Could you check a few things on this drawing? It's one solid part, dimensions in mm from its lowest x, y, z. A direction names the side the tool comes from. Round coordinates to 2 decimals unless told otherwise and drop trailing zeros. Loops run counter-clockwise (first coordinate to the right, second up) from the corner with the lowest first, then second, coordinate; pieces in that order, holes last. Notation, with made-up numbers: M 4,55 L 9,55 A6 ccw 9,66 Z; hole C 74,-35 d8. An arc over 180 degrees is marked long. Answer as a JSON object with one key per item and string values.
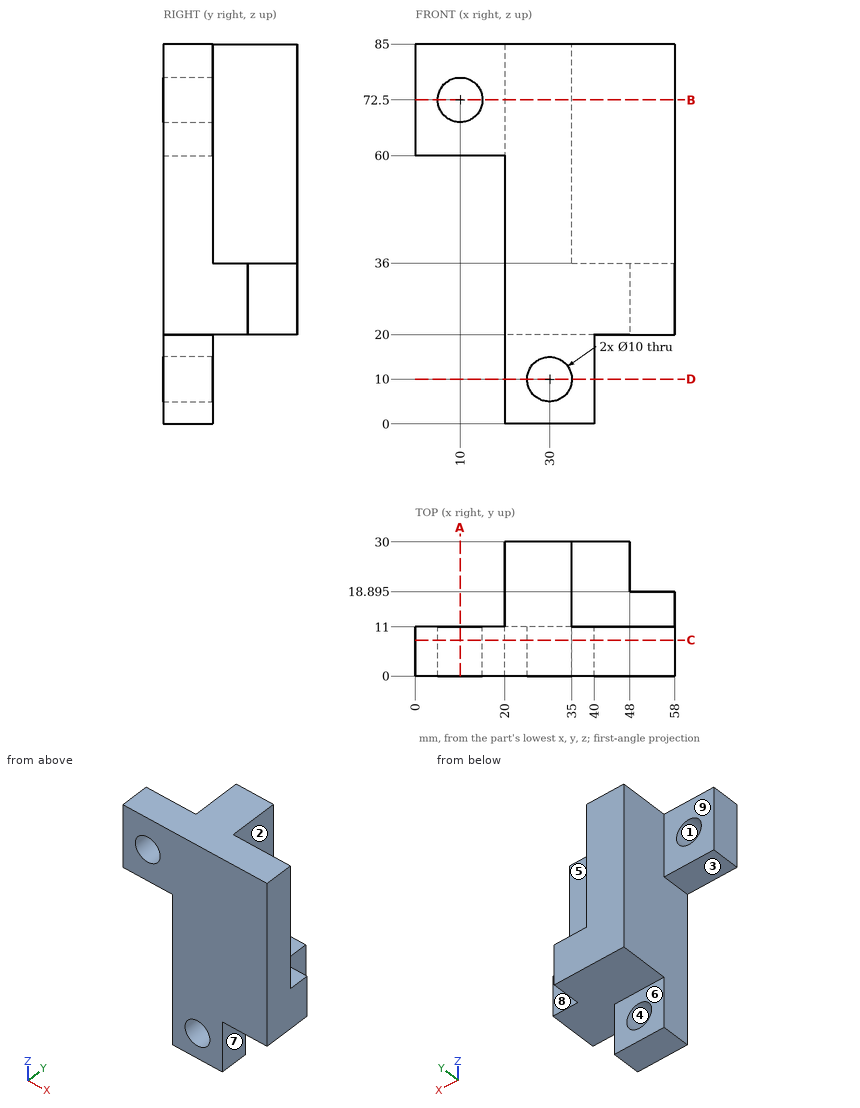
Item 1: I'm going to push flat-ended pins straight in: pin 1 Ø5.5 at (y, z) = (16, 71) entering from +X; pin 2 Ø15 at (x, y) = (48, 13) entering from -Z; pin 3 Ø11.5 at (x, z) = (48, 51.5) entering from +Y; pin 4 Ø6 at (x, z) = (9, 71.5) entering from +Y. Where does each tip first touch, or does it pass through?
Resolved:
{"pin 1": "x = 35", "pin 2": "z = 20", "pin 3": "y = 11", "pin 4": "through"}
Item 2: I want a section at B-B, the plane z = 72.5. Please give me the cut outline in (x, y), then the cut area to 3 significant figures.
Resolved:
{"outline": "M 0,0 L 5,0 L 5,11 L 0,11 Z; M 15,0 L 58,0 L 58,11 L 35,11 L 35,30 L 20,30 L 20,11 L 15,11 Z", "area": "813 mm²"}
Item 3: I want a section at A-A, the plane x = 10. Please give me the cut outline in (y, z).
Resolved:
{"outline": "M 0,60 L 11,60 L 11,67.5 L 0,67.5 Z; M 0,77.5 L 11,77.5 L 11,85 L 0,85 Z"}
Item 4: I want a section at D-D, the plane z = 10. Please give me the cut outline in (x, y), then the cut area to 3 significant figures.
Resolved:
{"outline": "M 20,0 L 25,0 L 25,11 L 20,11 Z; M 35,0 L 40,0 L 40,11 L 35,11 Z", "area": "110 mm²"}
Item 5: I want a section at C-C, the plane y = 8. Please give me the cut outline in (x, z).
Resolved:
{"outline": "M 0,60 L 20,60 L 20,0 L 40,0 L 40,20 L 58,20 L 58,85 L 0,85 Z; hole C 10,72.5 d10; hole C 30,10 d10"}
Item 6: On a 3-axis mill with a long thin cutter (end or side, diameter ignored), from which of +Z, -Z, +X, -X, +Y, -Y can I reach the whole of each face in a straight line? I mean the marked faces 5, 6, 7, 8 and 9. Say none if no direction works.
Resolved:
{"face 5": "+Z, +X, +Y", "face 6": "-Z, +X, -X, +Y", "face 7": "-Z, +X, +Y, -Y", "face 8": "+Z, -Z, +X, +Y", "face 9": "+Z, -Z, -X, +Y"}
Item 7: If we mould it in two halves opening along X, with no side actions, what happens to the marked faces 1, 2, 3 and 4? For each: pulls with the +X half, pulls with the -X half, needs draft (parallel to the pull), parting line crosses it, or undercut.
Resolved:
{"face 1": "undercut", "face 2": "pulls with the +X half", "face 3": "needs draft", "face 4": "undercut"}
Item 8: Please list where these lines run through material, in increasing order: probe 1 along Z at (x, y) = (10, 7); probe 2 along X at (y, z) = (6, 72.5); probe 3 along X at (y, z) = (8.5, 10). Write a range as from..to.
Resolved:
{"probe 1": "60..67.5, 77.5..85", "probe 2": "0..5, 15..58", "probe 3": "20..25, 35..40"}
